Input: part model. Units: mm. Frame: model coordinates. Coordinates: 2 decimals unless noted, no trailing zeros. Loops run counter-clockwise (first coordinate to the right, second up) from the corner with the lowest first, then second, coordinate; pieces in that order, holes last.
(1) Line query: L1, parallel to Z at x = -5, y = 2.05; L2, parallel to X at y = 0.2, z = -6.5; L3, parallel to Z at x = -3.8, y = 1.5. Output: solid intervals per line, ascending.
(2) Section B-B, the plane z = -3.25. Return loops of the section in (x, y) (3 decimals), then the cut area to 3 significant figures.
(3) Mould query, pull axis Z, two halves, no side actions, for faces 1 (the face through (-9.506, 1.565, 0.158)), 2 (the face through (-7, 3.175, 0)), 3 (the face through (-5.776, 1.565, 6.299)), 4 (the face through (-5.285, 1.565, -7.463)). Classes: released by +Z, released by -Z, zero draft, split by the parting line, or undercut.
(4) Contact query for flat-ended pins moving along their axis: P1, Ø1, axis at x = -6, y = 2.5, coming from the -Z side; P2, Ø1, axis at x = -5.15, z = 6.78, coming from the +Y side. Output: stop coordinate, or through.
(5) Section A-A, the plane y = 2.6. Return loops of the section in (x, z) (1 decimal), then the cut area to 3 significant figures.
(6) Section C-C, the plane x = -8.1. Return loops of the section in (y, z) (3 decimals).
```python
from build123d import *

# Parameters (mm, degrees)
F0_R     = 0.79375
F1_DEPTH = 3.175


with BuildPart() as f1:
    # F0 (on Front) → F1 (new body)
    with BuildSketch(Plane.XZ):
        with BuildLine():
            ThreePointArc((-3.9927783848, -5.5628118829), (-6.3316194647, 0.0440282554), (-4.0207951612, 5.6624733224))
            ThreePointArc((-4.0207951612, 5.6624733224), (-6.2658522276, 5.6568699137), (-6.2714555786, 7.9019269802))
            ThreePointArc((-6.2714555786, 7.9019269802), (-9.5066095757, 0.0361038994), (-6.2322320705, -7.8134722725))
            ThreePointArc((-6.2322320705, -7.8134722725), (-6.2378353965, -5.5684152606), (-3.9927783848, -5.5628118829))
        make_face()
        with BuildLine():
            ThreePointArc((-6.2714555786, 7.9019269802), (-6.2658522276, 5.6568699137), (-4.0207951612, 5.6624733224))
            ThreePointArc((-4.0207951612, 5.6624733224), (-3.6787096426, 6.176520959), (-3.5586253987, 6.7822001224))
            ThreePointArc((-3.5586253987, 6.7822001224), (-4.5404461975, 8.2496158629), (-6.2714555786, 7.9019269802))
        make_face()
        with Locations((-5.1461253987, 6.7822001224)):
            Circle(F0_R, mode=Mode.SUBTRACT)
        with BuildLine():
            ThreePointArc((-3.5250052017, -6.6881421035), (-3.6466057216, -6.0788023263), (-3.9927783848, -5.5628118829))
            ThreePointArc((-3.9927783848, -5.5628118829), (-6.2378353965, -5.5684152606), (-6.2322320705, -7.8134722725))
            ThreePointArc((-6.2322320705, -7.8134722725), (-4.5031654583, -8.1540415977), (-3.5250052017, -6.6881421035))
        make_face()
        with Locations((-5.1125052017, -6.6881421035)):
            Circle(F0_R, mode=Mode.SUBTRACT)
    extrude(amount=-F1_DEPTH)


solid = f1.part
```
Report:
1. L1: z = -8.27 to -7.47, -5.9 to -4.34, 4.46 to 6, 7.56 to 8.36
1. L2: x = -7.36 to -5.88, -4.34 to -3.54
1. L3: z = -7.58 to -5.8, 5.94 to 7.62
2. outline: (-9.001, 0) - (-5.607, 0) - (-5.607, 3.175) - (-9.001, 3.175) - close
2. area: 10.8 mm2
3. face 1: split by the parting line
3. face 2: zero draft
3. face 3: undercut
3. face 4: undercut
4. P1: stops at z = -8.23
4. P2: passes through
5. outline: (-6.3, 7.9) arc R11.1 ccw to (-6.2, -7.8) arc R1.6 ccw to (-4, -5.6) arc R7.9 cw to (-4, 5.7) arc R1.6 ccw to start; hole circle Ø1.6 at (-5.1, -6.7); hole circle Ø1.6 at (-5.1, 6.8)
5. area: 51.5 mm2
6. outline: (0, -5.348) - (3.175, -5.348) - (3.175, 5.475) - (0, 5.475) - close
